```python
from build123d import *

# Parameters (mm, degrees)
SKETCH1_R           = 28
BOSS_EXTRUDE1_DEPTH = 1
SKETCH2_W           = 5.602179168
SKETCH2_H           = 5.423853163
SKETCH2_W_2         = 5.409000575
SKETCH2_W_3         = 5.69543838
SKETCH2_H_2         = 5.43870575
BOSS_EXTRUDE3_DEPTH = 0.5
SKETCH3_R           = 1.87600115
SKETCH3_R_2         = 1.841544929
SKETCH3_R_3         = 1.880605589
BOSS_EXTRUDE4_DEPTH = 1


with BuildPart() as part:
    # Sketch1 → Boss-Extrude1 (new body)
    with BuildSketch(Plane(origin=(0, 0, 0), x_dir=(1, 0, 0), z_dir=(0, 1, 0))):
        with Locations(Location((0, 0, 0), (0, 0, 270))):
            Circle(SKETCH1_R)
    extrude(amount=BOSS_EXTRUDE1_DEPTH)

    # Sketch2 → Boss-Extrude3 (add)
    with BuildSketch(Plane(origin=(0, 1, 0), x_dir=(1, 0, 0), z_dir=(0, 1, 0))):
        Polygon((-8.980483261, 19.96365386), (-13.677677887, 17.251727279), (-16.47876747, 22.103356754), (-11.781572845, 24.815283336), align=None)
        with Locations((-23.714337206, -0.007426294)):
            Rectangle(SKETCH2_W, SKETCH2_H)
        with Locations((-11.737264504, -0.007426294)):
            Rectangle(SKETCH2_W_2, SKETCH2_H)
        Rectangle(SKETCH2_W_3, SKETCH2_H_2)
        Polygon((-10.441936471, 11.647258747), (-7.737436184, 6.96292684), (-3.040241558, 9.674853421), (-5.744741846, 14.359185329), align=None)
        Polygon((11.932764361, 18.259153573), (7.235569736, 20.971080154), (10.036659319, 25.82270963), (14.733853945, 23.110783048), align=None)
        Polygon((3.99982832, 15.366611623), (1.295328032, 10.682279715), (5.992522658, 7.970353134), (8.697022946, 12.654685041), align=None)
        with Locations((23.714337206, 2.007426294)):
            Rectangle(SKETCH2_W, SKETCH2_H)
        with Locations((11.737264504, 2.007426294)):
            Rectangle(SKETCH2_W_2, SKETCH2_H)
        Polygon((8.980483261, -17.96365386), (13.677677887, -15.251727279), (16.47876747, -20.103356754), (11.781572845, -22.815283336), align=None)
        Polygon((10.441936471, -9.647258747), (7.737436184, -4.96292684), (3.040241558, -7.674853421), (5.744741846, -12.359185329), align=None)
        Polygon((-11.932764361, -16.259153573), (-7.235569736, -18.971080154), (-10.036659319, -23.82270963), (-14.733853945, -21.110783048), align=None)
        Polygon((-3.99982832, -13.366611623), (-1.295328032, -8.682279715), (-5.992522658, -5.970353134), (-8.697022946, -10.654685041), align=None)
    extrude(amount=BOSS_EXTRUDE3_DEPTH)

    # Sketch3 → Boss-Extrude4 (add)
    with BuildSketch(Plane(origin=(0, 1.5, 0), x_dir=(1, 0, 0), z_dir=(0, 1, 0))):
        with Locations(Location((-23.895356308, 0, 0), (0, 0, 270))):
            Circle(SKETCH3_R)
        with Locations(Location((-11.523163477, 0, 0), (0, 0, 270))):
            Circle(SKETCH3_R_2)
        with Locations(Location((0, 0, 0), (0, 0, 270))):
            Circle(SKETCH3_R_3)
        with Locations(Location((-12.813703558, 21.193985595, 0), (0, 0, 270))):
            Circle(SKETCH3_R)
        with Locations(Location((-6.627607142, 10.479352303, 0), (0, 0, 270))):
            Circle(SKETCH3_R_2)
        with Locations(Location((11.08165275, 22.193985595, 0), (0, 0, 270))):
            Circle(SKETCH3_R)
        with Locations(Location((4.895556335, 11.479352303, 0), (0, 0, 270))):
            Circle(SKETCH3_R_2)
        with Locations(Location((23.895356308, 2, 0), (0, 0, 270))):
            Circle(SKETCH3_R)
        with Locations(Location((11.523163477, 2, 0), (0, 0, 270))):
            Circle(SKETCH3_R_2)
        with Locations(Location((12.813703558, -19.193985595, 0), (0, 0, 270))):
            Circle(SKETCH3_R)
        with Locations(Location((6.627607142, -8.479352303, 0), (0, 0, 270))):
            Circle(SKETCH3_R_2)
        with Locations(Location((-11.08165275, -20.193985595, 0), (0, 0, 270))):
            Circle(SKETCH3_R)
        with Locations(Location((-4.895556335, -9.479352303, 0), (0, 0, 270))):
            Circle(SKETCH3_R_2)
    extrude(amount=BOSS_EXTRUDE4_DEPTH)


solid = part.part
```
Work out the finished part from the listing and answer in its coordinate system (mm). A direction names the side the tool comes from. Give positions to 0.01 mm unless a question says otherwise; leave off trailing zeros. Order: outer loops, then holes, each group sorted by start corner. A loop starts at its lowest first (then second) coordinate and runs counter-clockwise, first axis right, second up. Notation, with made-up numbers: M -19,-4.5 L -4,-4.5 A36 ccw -4,34.5 Z; hole C -0.5,-22 d6. An arc over 180 degrees is marked long. Return JSON: item names as keys, results as strings.
1) A tool of negligible diameter and unlimited length cuts with its end or side. For faces 4 (the flat face through (7.326, 1.246, -10.28)), 5 (the cylindrical face through (-25.727, 1.993, -0.407)), 6 (the flat face through (-10.4, 1.25, -22.42)), from which of +Z, -Z, +X, -X, +Y, -Y can it reach the whole face along a straight path? Write none if from no direction.
Resolved:
{"face 4": "+X, +Y", "face 5": "+Y", "face 6": "-Z, +Y"}
2) For a pull along X with two mould halves and no side action, classify faces 1 (the flat face through (-9.11, 1.25, -9.34)), 2 (the flat face through (-11, 2.5, 0)), 3 (the flat face through (10.4, 1.25, 20.42)) as +X half, -X half, draft (parallel to the pull), parting line (faces both ways), or undercut.
Resolved:
{"face 1": "-X half", "face 2": "draft", "face 3": "undercut"}
3) Section A-A, the plane y = 1.9 is taken. Give the number of separate pieces and of enclosed holes in the cut face, plus the area to 3 significant figures.
Resolved:
{"separate pieces": "13", "enclosed holes": "0", "area": "141 mm^2"}
4) Section B-B, the plane x = 0 is taken. Write down the section's boundary in (y, z), plus the area to 3 significant figures.
Resolved:
{"outline": "M 0,-28 L 1,-28 L 1,-2.72 L 1.5,-2.72 L 1.5,-1.88 L 2.5,-1.88 L 2.5,1.88 L 1.5,1.88 L 1.5,2.72 L 1,2.72 L 1,28 L 0,28 Z", "area": "62.5 mm^2"}
5) Each of these flat-tipped pins is pushed along its axis until it touches: pin 1 (1 mm diameter, centred on y = 0.5, z = 11.5, fed in from +X); pin 2 (6 mm diameter, centred on x = -18, z = 10.5, fed in from +Y); pin 3 (0.6 mm diameter, centred on y = 1, z = -3.5, fed in from -X). Where does it stop, or does it pass through?
Resolved:
{"pin 1": "x = 25.75", "pin 2": "y = 1", "pin 3": "x = -27.82"}
6) Straight lines are drawn through the part: line 1 along Z through (x, y) = (-12.5, 2.1); line 2 along Y through (x, z) = (7, -14.5); line 3 along Z through (x, y) = (-12, 2.35). For each, find the intervals that lie inside material, in ascending order. Write a range as [from, to].
Resolved:
{"line 1": "[-23.04, -19.34], [-1.56, 1.56], [18.97, 21.42]", "line 2": "[0, 1]", "line 3": "[-22.88, -19.5], [-1.78, 1.78], [18.56, 21.83]"}
